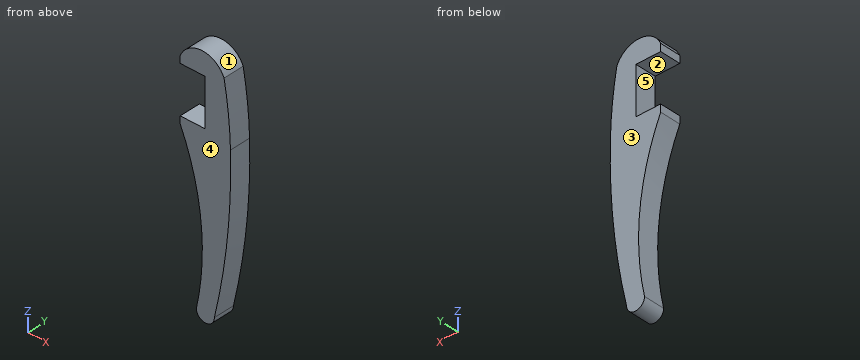
Autodesk Inventor part; units mm, degrees
ref_plane "YZ Plane" through (0, 0, 0) normal (1, 0, 0) x (0, 1, 0)
ref_plane "XZ Plane" through (0, 0, 0) normal (0, 1, 0) x (-1, 0, 0)
ref_plane "XY Plane" through (0, 0, 0) normal (0, 0, 1) x (1, 0, 0)
sketch "Sketch2" plane through (0, 0, 0) normal (0, 1, 0) x (-1, 0, 0)
  line L0 (0, 0) -> (11.8, 0)
  line L1 (11.8, 16.9404) -> (11.8, 22.5)
  line L2 (11.8, 22.5) -> (0, 22.5)
  line L3 (0, 22.5) -> (0, 0)
  arc A0 (-9.1414, 25.9755) -> (-12.2, -3.5) centre (181.3562, -8.6883) ccw
  arc A1 (11.8, 26) -> (-9.1414, 25.9755) centre (1.3346, 21.4702) ccw
  arc A2 (-4.4957, -79) -> (3.7221, -77.2478) centre (-0.2, -79) ccw
  arc A3 (-12.2, -3.5) -> (-4.4957, -79) centre (283.8313, -11.4351) ccw
  arc A4 (11.8, -3.5) -> (4.0957, -79) centre (122.1776, -52.9064) ccw
  line L4 (11.8, -3.5) -> (11.8, 0)
  line L5 (11.8, 22.5) -> (11.8, 26)
  dimension "d2" = 11.8
  dimension "d3" = 22.5
extrude "Extrusion1" add sketch "Sketch2" along normal blind 10 contours L0 L4 A4 A2 A3 A0 A1 L5 L2 L3
Part model, mm, in its own coordinate system. Face numbers are marked on the shaded views. A direction names the side the tool comes from. Coordinates: 2 decimals unless noted, no trailing zeros. Order: outer loops, then holes, each group sorted by start corner. A loop starts at its lowest first (then second) coordinate and runs counter-clockwise, first axis right, second up. Notation, with made-up numbers: (0, 87.5) - (49, 87.5) arc R19 cw to (49, 103.5) - close; hole circle Ø6 at (-3, 39.5). An arc over 180 degrees is marked (long way). Return JSON: item names as keys, results as strings. Group by question number.
Item 1: Drill centre lines: probe 1 along Z at (x, y) = (-10.5, 0.5); probe 2 along Z at (x, y) = (1.5, 0.5); probe 3 along X at (y, z) = (9, -27.5). Where is each one in solid material? Low to high. Write a range as from..to.
Item 2: Cut at C-C (z = -72). List the corners of the cut face in (x, y).
Item 3: Pull direction Z, two halves, no side cores. Call the marked faces 1, 2 and 3: pulls with the +Z half, pulls with the -Z half, needs draft (parallel to the pull), parting line crosses it, or undercut.
Item 4: Pin check, flat tips, straight feed: pin 1 (1 mm diameter, centred on y = 4, z = -34.5, fed in from -X); pin 2 (6 mm diameter, centred on x = -4.5, y = 8, fed in from -Z) (3 decimals); pin 3 (3 mm diameter, centred on y = 5, z = 9, fed in from -X). Stop position of each tip, or through.
Item 5: Cut at B-B (y = 1.25). List the corners of the cut face in (x, z).
Item 6: Which spindle directions (+Z, -Z, +X, -X, +Y, -Y) get a long thin tool onto all of the face, cutting with end or side? Do the marked faces 4 and 5. Say none if no direction does.
Item 7: Cut at A-A (x = -5.75). List the corners of the cut face in (y, z), plus the area to 3 significant figures.
Check values:
{
 "1": {"probe 1": "z = -6.51..0, 22.5..28.26", "probe 2": "z = -83.09..32.52", "probe 3": "x = -3.95..11.87"},
 "2": {"outline": "(-2.76, 0) - (6.05, 0) - (6.05, 10) - (-2.76, 10) - close"},
 "3": {"face 1": "pulls with the +Z half", "face 2": "undercut", "face 3": "needs draft"},
 "4": {"pin 1": "stops at x = -2.73", "pin 2": "stops at z = -82.945", "pin 3": "stops at x = 0"},
 "5": {"outline": "(-11.8, -3.5) arc R120.93 cw to (-4.1, -79) arc R4.3 ccw to (4.5, -79) arc R296.14 ccw to (12.2, -3.5) arc R193.63 ccw to (9.14, 25.98) arc R11.4 ccw to (-11.8, 26) - (-11.8, 22.5) - (0, 22.5) - (0, 0) - (-11.8, 0) - close"},
 "6": {"face 4": "+Z, -Z, +X, -X, -Y", "face 5": "-X, +Y, -Y"},
 "7": {"outline": "(0, -20.21) - (10, -20.21) - (10, 0) - (0, 0) - close; (0, 22.5) - (10, 22.5) - (10, 31.98) - (0, 31.98) - close", "area": "297 mm2"}
}
